Part model, mm, in its own coordinate system. Face numbers are marked on the shaded views. A direction names the side the tool comes from. Round coordinates to 2 decimals unless told otherwise and drop trailing zeros. Loops run counter-clockwise (first coordinate to the right, second up) from the corner with the lowest first, then second, coordinate; pieces in that order, holes last. Notation, with made-up numbers: (-33, -34.75) -> (13, -34.75) arc R21 ccw to (13, -1.75) -> close; hole circle Ø4 at (70.25, 34). An arc over 180 degrees is marked (long way). Use a Markdown table: item, result. Add a question column.
Item 1: Probe line 1 (Y direction, x = 0.75, z = -1.25); line 2 (Z direction, x = -0.5, y = -0.05); line 3 (X direction, y = 0.15, z = -1). List the from-to ranges inside material, lowest first. Write a range as [from, to].
Item 2: Cut at B-B, the plane z = -2.25. List the corners of the cut face in (x, y).
Item 3: Cut at A-A, the plane x = 0. List the corners of the cut face in (y, z).
Item 4: Which spindle directions (+Z, -Z, +X, -X, +Y, -Y) get a long thin tool onto all of the face, cutting with end or side? Do the marked faces 4 and 5. Say none if no direction does.
Item 5: Flat gauge pins, fed straight in: pin 1 (3 mm diameter, centred on x = 2, z = -6, fed in from -Y); pin 2 (0.6 mm diameter, centred on x = 0, y = 0, fed in from -Z); pin 3 (3 mm diameter, centred on x = -1, z = -5.5, fed in from +Y). Where does each tip first touch, or does it go through?
Item 6: Two-plate mould, pull along Y, no slides. Class the marked faces 1, 2 and 3: pulls with the +Y half, pulls with the -Y half, needs draft (parallel to the pull), parting line crosses it, or undercut.
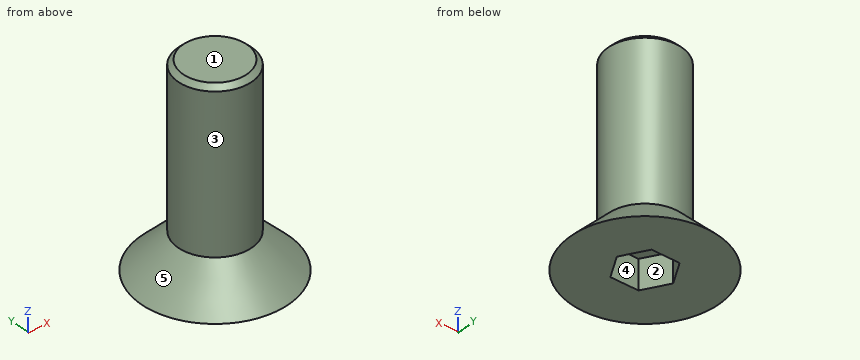
Autodesk Inventor part; units mm, degrees
ref_plane "YZ Plane" through (0, 0, 0) normal (1, 0, 0) x (0, 1, 0)
ref_plane "XZ Plane" through (0, 0, 0) normal (0, 1, 0) x (-1, 0, 0)
ref_plane "XY Plane" through (0, 0, 0) normal (0, 0, 1) x (1, 0, 0)
sketch "Sketch4" plane through (0, 0, 0) normal (1, 0, 0) x (0, 1, 0)
  line L0 (0, 0) -> (0, -8)
  line L1 (0, -8) -> (3, -8)
  line L2 (3, -8) -> (1.5, -6.5)
  line L3 (1.5, -6.5) -> (1.5, 0)
  line L4 (1.5, 0) -> (0, 0)
  dimension "d11" = 6
  dimension "d12" = 3
  dimension "d15" = 8
  dimension "d16" = 45
revolve "Revolution1" add sketch "Sketch4" angle 360 about axis through (0, 0, 0) along (0, 0, -1)
sketch "Sketch5" plane through (0, 0, -8) normal (0, 0, -1) x (-1, 0, 0)
  line L0 (1.1547, 0) -> (0.5774, -1)
  line L1 (0.5774, -1) -> (-0.5774, -1)
  line L2 (-0.5774, -1) -> (-1.1547, 0)
  line L3 (-1.1547, 0) -> (-0.5774, 1)
  line L4 (-0.5774, 1) -> (0.5774, 1)
  line L5 (0.5774, 1) -> (1.1547, 0)
  point P0 (0, 0)
  point P1 (0, 0)
  dimension "d18" = 2
extrude "Extrusion5" cut sketch "Sketch5" against normal blind 1.2
chamfer "Chamfer2" distance 0.2 angle 45 1 edges at (0, -1.5, 0)
thread "Thread1"
properties part number "M3 x 8mm FHCS" material "Stainless Steel"
A:
| question | item | result |
|---|---|---|
| 1 | line 1 | y = [-1.3, 1.3] |
| 1 | line 2 | z = [-6.8, 0] |
| 1 | line 3 | x = [-1.49, 1.49] |
| 2 | outline | circle Ø3 at (0, 0) |
| 3 | outline | (-3, -8) -> (-1, -8) -> (-1, -6.8) -> (1, -6.8) -> (1, -8) -> (3, -8) -> (1.5, -6.5) -> (1.5, -0.2) -> (1.3, 0) -> (-1.3, 0) -> (-1.5, -0.2) -> (-1.5, -6.5) -> close |
| 4 | face 4 | -Z |
| 4 | face 5 | +Z |
| 5 | pin 1 | stops at y = -1.93 |
| 5 | pin 2 | stops at z = -6.8 |
| 5 | pin 3 | stops at y = 1.85 |
| 6 | face 1 | needs draft |
| 6 | face 2 | undercut |
| 6 | face 3 | parting line crosses it |
